Read the model definition and answer for the solid it produces. Units are mm, in the model's axes. Face numbers are marked on the shaded views. A direction names the side the tool comes from. Give positions to 0.01 mm unless a question says otherwise; leave off trailing zeros. Loops run counter-clockwise (first coordinate to the right, second up) from the corner with the lowest first, then second, coordinate; pieces in that order, holes last. Notation, with made-up numbers: (21.25, 67) -> (57.25, 67) arc R16 cw to (57.25, 74) -> close; hole circle Ø3 at (53, 64.25). An arc over 180 degrees is marked (long way). Answer as CSV lines item,"result". Start each with the question number.
```python
from build123d import *

# Parameters (mm, degrees)
SKETCH1_R           = 3
BOSS_EXTRUDE1_DEPTH = 5
SKETCH2_R           = 12
CUT_EXTRUDE1_DEPTH  = 5
SKETCH2_3_R         = 16
SKETCH2_3_R_2       = 12
BOSS_EXTRUDE2_DEPTH = 13
BOSS_EXTRUDE5_DEPTH = 4.5


with BuildPart() as part:
    # Sketch1 → Boss-Extrude1 (new body)
    with BuildSketch(Plane(origin=(0, 0, 0), x_dir=(1, 0, 0), z_dir=(0, 1, 0))):
        with BuildLine():
            Line((-60, 32), (60, 32))
            ThreePointArc((60, 32), (64.242640687, 30.242640687), (66, 26))
            Line((66, 26), (66, -26))
            ThreePointArc((66, -26), (64.242640687, -30.242640687), (60, -32))
            Line((60, -32), (-60, -32))
            ThreePointArc((-60, -32), (-64.242640687, -30.242640687), (-66, -26))
            Line((-66, -26), (-66, 26))
            ThreePointArc((-66, 26), (-64.242640687, 30.242640687), (-60, 32))
        make_face()
        with Locations((-60, 26)):
            Circle(SKETCH1_R, mode=Mode.SUBTRACT)
        with Locations((-60, -26)):
            Circle(SKETCH1_R, mode=Mode.SUBTRACT)
        with Locations((60, 26)):
            Circle(SKETCH1_R, mode=Mode.SUBTRACT)
        with Locations((60, -26)):
            Circle(SKETCH1_R, mode=Mode.SUBTRACT)
    extrude(amount=BOSS_EXTRUDE1_DEPTH)

    # Sketch2 → Cut-Extrude1 (cut)
    with BuildSketch(Plane(origin=(0, 5, 0), x_dir=(1, 0, 0), z_dir=(0, 1, 0))):
        Circle(SKETCH2_R)
    extrude(amount=-CUT_EXTRUDE1_DEPTH, mode=Mode.SUBTRACT)

    # Sketch2_3 → Boss-Extrude2 (add)
    with BuildSketch(Plane(origin=(0, 5, 0), x_dir=(1, 0, 0), z_dir=(0, 1, 0))):
        Circle(SKETCH2_3_R)
        Circle(SKETCH2_3_R_2, mode=Mode.SUBTRACT)
    extrude(amount=BOSS_EXTRUDE2_DEPTH)

    # Sketch4 → Boss-Extrude5 (add, symmetric)
    with BuildSketch(Plane(origin=(0, 0, 0), x_dir=(0.866025404, 0, -0.5), z_dir=(0.5, 0, 0.866025404))):
        Polygon((-45, 5), (-14.70481954, 14.843500832), (-14.70481954, 5), align=None)
        Polygon((14.70481954, 14.843500832), (14.70481954, 5), (45, 5), align=None)
    boss_extrude5 = extrude(amount=BOSS_EXTRUDE5_DEPTH, both=True)

    # Mirror1: Boss-Extrude5 across plane
    add(boss_extrude5.mirror(Plane.XY))


solid = part.part
```
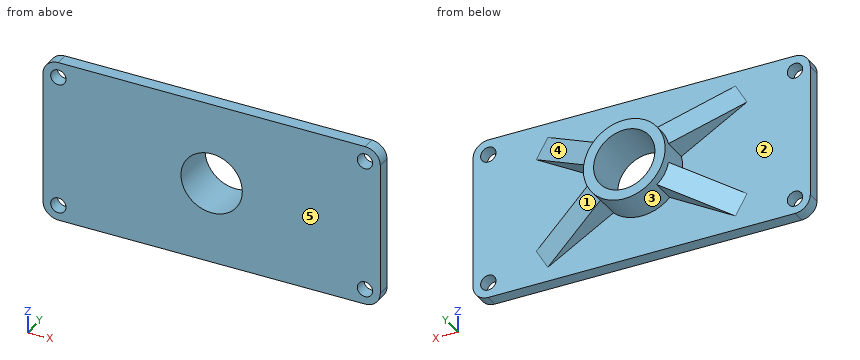
(1) Find section D-D on x = 49. Write down the section's boundary in (y, z).
(2) Find the intervals of material crossed by line 1 along X through (y, z) = (3.3, -26); line 2 along Z through (x, y) = (-60, 4.05); line 3 along Z through (x, y) = (0, 12.75), in increasing order. Write a range as from..to.
(3) A tool of negligible diameter and unlimited length cuts with its end or side. For the marked faces 1 and 2, from which of +Z, -Z, +X, -X, +Y, -Y can it reach the whole face along a straight path? Write none if from no direction.
(4) Find section B-B on y = 11.5. Write down the section's boundary in (x, z).
(5) Find section A-A on x = 0. Write down the section's boundary in (y, z), then the cut area to 3 significant figures.
(6) Each of these flat-tipped pins is pushed along its axis until it touches: P1, Ø2, axis at x = -24, y = 7, coming from the -Z side; P2, Ø1.5, axis at x = -5, y = 10.5, coming from the -Z side; P3, Ø3.5, axis at x = 60, z = -26, coming from the -Y side; P4, Ø12, axis at x = 42, z = -3, coming from the +Y side. Where does it stop, or does it pass through?
(7) Find section C-C on x = -30. Write down the section's boundary in (y, z).
(8) The mould has two halves that part along X. Classify the marked faces 3, 4 and 5: pulls with the +X half, pulls with the -X half, needs draft (parallel to the pull), parting line crosses it, or undercut.
Answer block:
1,outline,"(0, -32) -> (5, -32) -> (5, 32) -> (0, 32) -> close"
2,line 1,"x = -66..-63, -57..57, 63..66"
2,line 2,"z = -32..-29, -23..23, 29..32"
2,line 3,"z = -16..-12, 12..16"
3,face 1,"-Z, +X, +Y"
3,face 2,"+Y"
4,outline,"(-23.9, -8.6) -> (-19.4, -16.39) -> (-11.05, -11.57) arc R16 ccw to (11.05, -11.57) -> (19.4, -16.39) -> (23.9, -8.6) -> (15.55, -3.78) arc R16 ccw to (15.55, 3.78) -> (23.9, 8.6) -> (19.4, 16.39) -> (11.05, 11.57) arc R16 ccw to (-11.05, 11.57) -> (-19.4, 16.39) -> (-23.9, 8.6) -> (-15.55, 3.78) arc R16 ccw to (-15.55, -3.78) -> close; hole circle Ø24 at (0, 0)"
5,outline,"(0, -32) -> (5, -32) -> (5, -16) -> (18, -16) -> (18, -12) -> (0, -12) -> close; (0, 12) -> (18, 12) -> (18, 16) -> (5, 16) -> (5, 32) -> (0, 32) -> close"
5,area,"304 mm2"
6,P1,"stops at z = -19.63"
6,P2,"stops at z = -15.43"
6,P3,"passes through"
6,P4,"stops at y = 5"
7,outline,"(0, -32) -> (5, -32) -> (5, -22.52) -> (7.52, -22.52) -> (9.21, -12.12) -> (5, -12.12) -> (5, 12.12) -> (9.21, 12.12) -> (7.52, 22.52) -> (5, 22.52) -> (5, 32) -> (0, 32) -> close"
8,face 3,"undercut"
8,face 4,"pulls with the +X half"
8,face 5,"needs draft"
